```python
from build123d import *

# Parameters (mm, degrees)
BOSS_EXTRUDE1_DEPTH   = 7.62
BOSS_EXTRUDE1_2_DEPTH = 7.62
BOSS_EXTRUDE1_3_DEPTH = 7.62
BOSS_EXTRUDE1_4_DEPTH = 7.62
SKETCH2_W             = 165.1
SKETCH2_H             = 20
BOSS_EXTRUDE2_DEPTH   = 6.35
LPATTERN2_COUNT       = 2
LPATTERN2_PITCH       = 82.55
CUT_EXTRUDE1_DEPTH    = 157.048617104
FILLET1_R             = 2.54
SKETCH6_W             = 25.4
SKETCH6_H             = 25.4
BOSS_EXTRUDE7_DEPTH   = 12.7
FILLET3_R             = 7.62
FILLET5_R             = 7.62
SKETCH11_R            = 1.984375
CUT_EXTRUDE3_DEPTH    = 169.09345118
SKETCH13_R            = 3.5
CUT_EXTRUDE5_DEPTH    = 159.282684864
FILLET6_R             = 2.54


with BuildPart() as part:
    # Sketch1 → Boss-Extrude1 (new body)
    with BuildSketch(Plane(origin=(0, 0, 0), x_dir=(1, 0, 0), z_dir=(0, 1, 0))):
        Polygon((-2.9718, 10), (-2.9718, 7.714), (-4.4450054, 7.714), (-4.4450054, 6.444), (-2.9718, 4.158), (2.9718, 4.158), (4.4449946, 6.444), (4.4449946, 7.714), (2.9718, 7.714), (2.9718, 10), align=None)
    boss_extrude1 = extrude(amount=BOSS_EXTRUDE1_DEPTH)



with BuildPart() as body_2:
    # Sketch1 → Boss-Extrude1 2 (new body)
    with BuildSketch(Plane(origin=(0, 0, 0), x_dir=(1, 0, 0), z_dir=(0, 1, 0))):
        Polygon((4.158, -2.9718), (4.158, 2.9718), (6.444, 4.4449946), (7.714, 4.4449946), (7.714, 2.9718), (10, 2.9718), (10, -2.9718), (7.714, -2.9718), (7.714, -4.4450054), (6.444, -4.4450054), align=None)
    boss_extrude1_2 = extrude(amount=BOSS_EXTRUDE1_2_DEPTH)


with BuildPart() as body_3:
    # Sketch1 → Boss-Extrude1 3 (new body)
    with BuildSketch(Plane(origin=(0, 0, 0), x_dir=(1, 0, 0), z_dir=(0, 1, 0))):
        Polygon((4.4450054, -6.444), (2.9718, -4.158), (-2.9718, -4.158), (-4.4449946, -6.444), (-4.4449946, -7.714), (-2.9718, -7.714), (-2.9718, -10), (2.9718, -10), (2.9718, -7.714), (4.4450054, -7.714), align=None)
    boss_extrude1_3 = extrude(amount=BOSS_EXTRUDE1_3_DEPTH)


with BuildPart() as body_4:
    # Sketch1 → Boss-Extrude1 4 (new body)
    with BuildSketch(Plane(origin=(0, 0, 0), x_dir=(1, 0, 0), z_dir=(0, 1, 0))):
        Polygon((-10, -2.9718), (-10, 2.9718), (-7.714, 2.9718), (-7.714, 4.4450054), (-6.444, 4.4450054), (-4.158, 2.9718), (-4.158, -2.9718), (-6.444, -4.4449946), (-7.714, -4.4449946), (-7.714, -2.9718), align=None)
    boss_extrude1_4 = extrude(amount=BOSS_EXTRUDE1_4_DEPTH)


with BuildPart() as part_1:
    add(part.part)

    add(body_2.part)  # Boss-Extrude2 merges body 2

    add(body_3.part)  # Boss-Extrude2 merges body 3

    add(body_4.part)  # Boss-Extrude2 merges body 4
    # Sketch2 → Boss-Extrude2 (add)
    with BuildSketch(Plane.XZ):
        with Locations((-72.55, 0)):
            Rectangle(SKETCH2_W, SKETCH2_H)
    extrude(amount=BOSS_EXTRUDE2_DEPTH)

    # LPattern2: Boss-Extrude1, Boss-Extrude1 2, Boss-Extrude1 3, Boss-Extrude1 4 ×2
    with Locations(*[(-i * LPATTERN2_PITCH, 0, 0) for i in range(1, LPATTERN2_COUNT)]):
        add(boss_extrude1)
        add(boss_extrude1_2)
        add(boss_extrude1_3)
        add(boss_extrude1_4)

    # Sketch4 → Cut-Extrude1 (cut, through all)
    with BuildSketch(Plane(origin=(0, -6.35, 0), x_dir=(-1, 0, 0), z_dir=(0, -1, 0))):
        Polygon((155.1, -10), (117.5588, -10), (155.1, -0.2108), align=None)
    extrude(amount=-CUT_EXTRUDE1_DEPTH, mode=Mode.SUBTRACT)

    # Fillet1
    fillet1_edges = [part_1.edges().sort_by_distance(p)[0] for p in [
        (-117.5588, -3.175, 10),
    ]]
    fillet(fillet1_edges, radius=FILLET1_R)

    # Sketch6 → Boss-Extrude7 (add)
    with BuildSketch(Plane.ZY.offset(155.1)):
        with Locations((-12.4892, 6.35)):
            Rectangle(SKETCH6_W, SKETCH6_H)
    extrude(amount=-BOSS_EXTRUDE7_DEPTH)

    # Fillet3
    fillet3_edges = [part_1.edges().sort_by_distance(p)[0] for p in [
        (-142.4, 0, -4.8946),
        (-142.4, -3.175, -10),
    ]]
    fillet(fillet3_edges, radius=FILLET3_R)

    # Fillet5
    # the kernel refuses this fillet: 7.62 mm, written as the material it takes off along each edge
    with BuildSketch(Plane(origin=(-142.4, 38.1, 0.2108), x_dir=(-1, 0, 0), z_dir=(0, -1, 0))) as fillet5_piece_1:
        with BuildLine():
            CenterArc((FILLET5_R, FILLET5_R), FILLET5_R, 180, 90)
            Line((0, FILLET5_R), (0, 0))
            Line((0, 0), (FILLET5_R, 0))
        make_face()
    extrude(amount=30.48, mode=Mode.SUBTRACT)
    with BuildSketch(Plane(origin=(-134.78, 7.62, 0.2108), x_dir=(0.5976672776328269, 0.8017442392976487, 0), z_dir=(-0.8017442392976487, 0.5976672776328269, 0))) as fillet5_piece_2_section:
        with BuildLine():
            CenterArc((7.62 + FILLET5_R, FILLET5_R), FILLET5_R, 180, 90)
            Line((7.62, FILLET5_R), (7.62, 0))
            Line((7.62, 0), (7.62 + FILLET5_R, 0))
        make_face()
    fillet5_piece_2 = revolve(axis=Axis((-134.78, 7.62, 0.2108), (0, 0, -1)), revolution_arc=233.296989237, mode=Mode.PRIVATE)
    fillet5_piece_2 = split(fillet5_piece_2, bisect_by=Plane(origin=(-140.494534821, 0, -2.163807691), z_dir=(0, 1, 0)), keep=Keep.TOP, mode=Mode.PRIVATE)
    add(fillet5_piece_2, mode=Mode.SUBTRACT)

    # Sketch11 → Cut-Extrude3 (cut, through all)
    with BuildSketch(Plane.ZY.offset(155.1)):
        with Locations((-12.4892, 6.35)):
            Circle(SKETCH11_R)
    extrude(amount=-CUT_EXTRUDE3_DEPTH, mode=Mode.SUBTRACT)

    # Sketch13 → Cut-Extrude5 (cut, through all)
    with BuildSketch(Plane(origin=(0, 0, 0), x_dir=(1, 0, 0), z_dir=(0, 1, 0))):
        with Locations(Location((0, 0, 0), (0, 0, 270))):
            Circle(SKETCH13_R)
        with Locations(Location((-82.55, 0, 0), (0, 0, 270))):
            Circle(SKETCH13_R)
    extrude(amount=-CUT_EXTRUDE5_DEPTH, mode=Mode.SUBTRACT)

    # Fillet6
    fillet6_edges = [part_1.edges().sort_by_distance(p)[0] for p in [
        (0, -6.35, -3.5),
        (-82.55, -6.35, -3.5),
    ]]
    fillet(fillet6_edges, radius=FILLET6_R)


solid = part_1.part
```
Here's how the part is built. I have some questions about the finished solid (model axes, mm). A direction names the side the tool comes from. Round coordinates to 2 decimals unless told otherwise and drop trailing zeros. Order: outer loops, then holes, each group sorted by start corner. A loop starts at its lowest first (then second) coordinate and runs counter-clockwise, first axis right, second up. Notation, with made-up numbers: (82.5, 38) -> (86.5, 38) arc R18 ccw to (86.5, 45) -> close; hole circle Ø6 at (-3.5, 38.5). An arc over 180 degrees is marked (long way). Use a Markdown table: item, result. Add a question column.
(1) Suppose I cut it at C-C, the plane x = -106.5. Please give me the cut outline in (y, z), and give its area (3 significant figures).
(2) Suppose I cut it at B-B, the plane z = -16. Please give me the cut outline in (x, y), and give its area (3 significant figures).
(3) For faces 4 (the face through (4.158, 4, 0)), 5 (the face through (-75, 7.62, 0)), 6 (the face through (-63, -2, -10)), which set-ups out of +Z, -Z, +X, -X, +Y, -Y let a thin tool reach every point of the face, with its end or its side?
(4) For pin 1 Ø1.5 at (x, y) = (-76, 0.5) entering from +Z; pin 2 Ø1.4 at (y, z) = (2.5, 7) entering from +X (3 decimals); pin 3 Ø1 at (x, y) = (-86.5, 10) entering from -Z; pin 4 Ø4.5 at (x, z) = (-76, 1) entering from +Y, each with a flat end and sliding along its axis, tell me the tip position at first contact or that it passes through.
(5) I need wall thicknesses on line 1 along X through (y, z) = (-1.2, 0); line 2 along X through (y, z) = (2, 5); line 3 along Y through (x, z) = (-112.5, -3.5). Which ranges of each line are inside material? Lowest first, please.
(6) If we mould it in two halves opening along Y, with no side actions, what happens to faces 1 (the face through (-78.392, 4, 0)), 2 (the face through (-148.479, 5.59, -10.656)), 3 (the face through (-83, 7.62, 7))? For each: released by +Y, released by -Y, zero draft, split by the parting line, or undercut.
(7) Suppose I cut it at A-A, the plane x = 0. Please give me the cut outline in (y, z).
Verdict:
| question | item | result |
|---|---|---|
| 1 | outline | (-6.35, -10) -> (0, -10) -> (0, 10) -> (-6.35, 10) -> close |
| 1 | area | 127 mm2 |
| 2 | outline | (-155.1, -6.35) -> (-142.23, -6.35) -> (-142.23, 6) arc R7.62 cw to (-142.4, 7.62) -> (-142.4, 19.05) -> (-155.1, 19.05) -> close |
| 2 | area | 325 mm2 |
| 3 | face 4 | +Y |
| 3 | face 5 | +Z, -Z, +X, +Y |
| 3 | face 6 | -Z, +X, +Y, -Y |
| 4 | pin 1 | z = 10 |
| 4 | pin 2 | x = 4.445 |
| 4 | pin 3 | through |
| 4 | pin 4 | y = 7.62 |
| 5 | line 1 | -155.1 to -86.05, -79.05 to -3.5, 3.5 to 10 |
| 5 | line 2 | -86.06 to -79.04, -3.51 to 3.51 |
| 5 | line 3 | -6.35 to 0 |
| 6 | face 1 | zero draft |
| 6 | face 2 | undercut |
| 6 | face 3 | released by +Y |
| 7 | outline | (-6.35, -10) -> (7.62, -10) -> (7.62, -4.16) -> (0, -4.16) -> (0, -3.5) -> (-3.81, -3.5) arc R2.54 ccw to (-6.35, -6.04) -> close; (-6.35, 6.04) arc R2.54 ccw to (-3.81, 3.5) -> (0, 3.5) -> (0, 4.16) -> (7.62, 4.16) -> (7.62, 10) -> (-6.35, 10) -> close |
